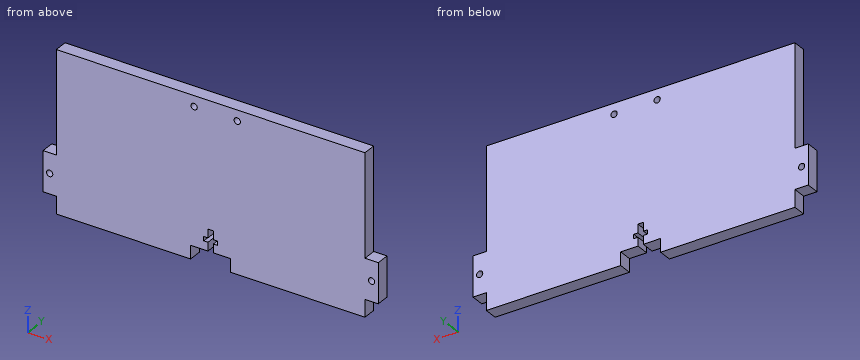
```python
from build123d import *

# Parameters (mm, degrees)
SKETCH1_R           = 1.5
BOSS_EXTRUDE1_DEPTH = 6.35
SKETCH2_R           = 1.5
CUT_EXTRUDE1_DEPTH  = 7.35
CUT_EXTRUDE2_DEPTH  = 7.35


with BuildPart() as part:
    # Sketch1 → Boss-Extrude1 (new body)
    with BuildSketch(Plane(origin=(0, 0, 0), x_dir=(1, 0, 0), z_dir=(0, 1, 0))):
        Polygon((-73.66, -34.925), (73.66, -34.925), (73.66, 13.97), (80.01, 13.97), (80.01, 33.02), (73.66, 33.02), (73.66, 34.925), (73.66, 41.275), (9.525, 41.275), (9.525, 34.925), (-9.525, 34.925), (-9.525, 41.275), (-73.66, 41.275), (-73.66, 34.925), (-73.66, 33.02), (-80.01, 33.02), (-80.01, 13.97), (-73.66, 13.97), align=None)
        with Locations((-76.835, 23.495)):
            Circle(SKETCH1_R, mode=Mode.SUBTRACT)
        with Locations((76.835, 23.495)):
            Circle(SKETCH1_R, mode=Mode.SUBTRACT)
    extrude(amount=BOSS_EXTRUDE1_DEPTH)

    # Sketch2 → Cut-Extrude1 (cut, through all)
    with BuildSketch(Plane(origin=(0, 6.35, 0), x_dir=(1, 0, 0), z_dir=(0, 1, 0))):
        with Locations((12.7, -29.845)):
            Circle(SKETCH2_R)
        with Locations((-7.874, -29.845)):
            Circle(SKETCH2_R)
    extrude(amount=-CUT_EXTRUDE1_DEPTH, mode=Mode.SUBTRACT)

    # Sketch3 → Cut-Extrude2 (cut, through all)
    with BuildSketch(Plane(origin=(0, 6.35, 0), x_dir=(1, 0, 0), z_dir=(0, 1, 0))):
        Polygon((-1.27, 34.925), (1.27, 34.925), (1.27, 30.861), (3.302, 30.861), (3.302, 28.829), (1.27, 28.829), (1.27, 24.765), (-1.27, 24.765), (-1.27, 28.829), (-3.302, 28.829), (-3.302, 30.861), (-1.27, 30.861), align=None)
    extrude(amount=-CUT_EXTRUDE2_DEPTH, mode=Mode.SUBTRACT)


solid = part.part
```
Work out the finished part from the listing and answer in its coordinate system (mm). Round coordinates to 2 decimals unless told otherwise and drop trailing zeros. Write each loop counter-clockwise with the first axis right and the second up, starting at its lowest first coordinate (ties: lowest second). Pieces come first, ordered by that corner, then holes. Notation, with made-up numbers: (26, -18.5) - (37, -18.5) arc R20 cw to (37, -12.5) - close; hole circle Ø2 at (20, 78.5). An arc over 180 degrees is marked (long way). Return JSON: item names as keys, results as strings. Group by question number.
Q1. The part is cut by section B-B on y = 1.5. Count the separate pieces of the cut face and the enclosed holes in it, then the cut area to 3 significant figures.
Q2. The part is cut by section C-C on z = 11. Write down the section's boundary in (x, y).
Q3. Each of these flat-tipped pins is pushed along its axis until it touches: pin 1 Ø1.3 at (x, y) = (0.5, 4) entering from -Z (3 decimals); pin 2 Ø0.6 at (x, y) = (-2, 3) entering from -Z (3 decimals); pin 3 Ø1.9 at (x, y) = (-77, 3) entering from -Z; pin 4 Ø4 at (x, z) = (76.835, -23.495) entering from +Y. Where does it stop, or does it pass through?
Q4. Find the intervals of material crossed by L1, parallel to X at y = 3, z = -24; L2, parallel to Z at x = 12.7, y = 3.5 (3 decimals); L3, parallel to X at y = 3.25, z = -26, in increasing order.
Q5. The part is cut by section A-A on x = 12.7. Write down the section's boundary in (y, z) (3 decimals).
Solved:
{
 "1": {"separate pieces": "1", "enclosed holes": "4", "area": "11,300 mm²"},
 "2": {"outline": "(-73.66, 0) - (73.66, 0) - (73.66, 6.35) - (-73.66, 6.35) - close"},
 "3": {"pin 1": "z = -24.765", "pin 2": "z = -34.925", "pin 3": "z = -33.02", "pin 4": "y = 6.35"},
 "4": {"L1": "-80.01 to -78.25, -75.42 to 75.42, 78.25 to 80.01", "L2": "-41.275 to 28.345, 31.345 to 34.925", "L3": "-80.01 to -1.27, 1.27 to 80.01"},
 "5": {"outline": "(0, -41.275) - (6.35, -41.275) - (6.35, 28.345) - (0, 28.345) - close; (0, 31.345) - (6.35, 31.345) - (6.35, 34.925) - (0, 34.925) - close"}
}
